from build123d import *

# Parameters (mm, degrees)
SKETCH_1_W          = 20
SKETCH_1_H          = 60
EXTRUDE_1_DEPTH     = 7
SKETCH_4_W          = 30
SKETCH_4_H          = 32
EXTRUDE_2_DEPTH     = 7
SKETCH_3_W          = 9.8
SKETCH_3_H          = 45.5
CUT_EXTRUDE_1_DEPTH = 5
SKETCH_5_W          = 3.5
SKETCH_5_H          = 35
CUT_EXTRUDE_2_DEPTH = 34.911649916
SKETCH_6_R          = 1.1
CUT_EXTRUDE_3_DEPTH = 34.911649916
SKETCH_7_R          = 1.15
CUT_EXTRUDE_4_DEPTH = 35.263683398
FILLET_1_R          = 3
SKETCH_8_R          = 1.95
CUT_EXTRUDE_5_DEPTH = 1


with BuildPart() as part:
    # 草图1 → 凸台-拉伸1 (new body)
    with BuildSketch(Plane(origin=(0, 0, 0), x_dir=(1, 0, 0), z_dir=(0, 1, 0))):
        Rectangle(SKETCH_1_W, SKETCH_1_H)
    extrude(amount=EXTRUDE_1_DEPTH)

    # 草图4 → 凸台-拉伸2 (add)
    with BuildSketch(Plane.XZ):
        with Locations((0, 14)):
            Rectangle(SKETCH_4_W, SKETCH_4_H)
    extrude(amount=-EXTRUDE_2_DEPTH)

    # 草图3 → 切除-拉伸1 (cut)
    with BuildSketch(Plane(origin=(0, 7, 0), x_dir=(1, 0, 0), z_dir=(0, 1, 0))):
        with Locations((0, 2.25)):
            Rectangle(SKETCH_3_W, SKETCH_3_H)
    extrude(amount=-CUT_EXTRUDE_1_DEPTH, mode=Mode.SUBTRACT)

    # 草图5 → 切除-拉伸2 (cut, through all)
    with BuildSketch(Plane(origin=(0, 2, 0), x_dir=(1, 0, 0), z_dir=(0, 1, 0))):
        with Locations((0, 2.25)):
            Rectangle(SKETCH_5_W, SKETCH_5_H)
    extrude(amount=-CUT_EXTRUDE_2_DEPTH, mode=Mode.SUBTRACT)

    # 草图6 → 切除-拉伸3 (cut, through all)
    with BuildSketch(Plane(origin=(0, 2, 0), x_dir=(1, 0, 0), z_dir=(0, 1, 0))):
        with Locations(Location((0, 22.75, 0), (0, 0, 270))):
            Circle(SKETCH_6_R)
        with Locations(Location((0, -18.25, 0), (0, 0, 90))):
            Circle(SKETCH_6_R)
    extrude(amount=-CUT_EXTRUDE_3_DEPTH, mode=Mode.SUBTRACT)

    # 草图7 → 切除-拉伸4 (cut, through all)
    with BuildSketch(Plane(origin=(0, 7, 0), x_dir=(1, 0, 0), z_dir=(0, 1, 0))):
        with Locations(Location((-12, -1, 0), (0, 0, 270))):
            Circle(SKETCH_7_R)
        with Locations(Location((12, -1, 0), (0, 0, 90))):
            Circle(SKETCH_7_R)
        with Locations(Location((12, -27, 0), (0, 0, 270))):
            Circle(SKETCH_7_R)
        with Locations(Location((-12, -27, 0), (0, 0, 90))):
            Circle(SKETCH_7_R)
    extrude(amount=-CUT_EXTRUDE_4_DEPTH, mode=Mode.SUBTRACT)

    # 圆角1
    fillet_1_edges = [part.edges().sort_by_distance(p)[0] for p in [
        (10, 3.5, -2),
        (-10, 3.5, -2),
    ]]
    fillet(fillet_1_edges, radius=FILLET_1_R)

    # 草图8 → 切除-拉伸5 (cut)
    with BuildSketch(Plane.XZ):
        with Locations(Location((0, 18.25, 0), (0, 0, 270))):
            Circle(SKETCH_8_R)
        with Locations(Location((0, -22.75, 0), (0, 0, 270))):
            Circle(SKETCH_8_R)
    extrude(amount=-CUT_EXTRUDE_5_DEPTH, mode=Mode.SUBTRACT)


solid = part.part
CAD build for the part. Positions are in the model's coordinates, mm. A direction names the side the tool comes from. Round coordinates to 2 decimals unless told otherwise and drop trailing zeros. Loops run counter-clockwise (first coordinate to the right, second up) from the corner with the lowest first, then second, coordinate; pieces in that order, holes last. Notation, with made-up numbers: (53, -36) - (106, -36) arc R19 ccw to (106, -9) - close; hole circle Ø4 at (83.25, -31.75). An arc over 180 degrees is marked (long way). Put each result on its own line as item: value.
1. Slice it at B-B on x = 0. List the corners of the cut face in (y, z), and give its area (3 significant figures).
Geometry check:
outline: (0, -30) - (7, -30) - (7, -25) - (2, -25) - (2, -23.85) - (1, -23.85) - (1, -24.7) - (0, -24.7) - close; (0, -20.8) - (1, -20.8) - (1, -21.65) - (2, -21.65) - (2, -19.75) - (0, -19.75) - close; (0, 15.25) - (2, 15.25) - (2, 17.15) - (1, 17.15) - (1, 16.3) - (0, 16.3) - close; (0, 20.2) - (1, 20.2) - (1, 19.35) - (2, 19.35) - (2, 20.5) - (7, 20.5) - (7, 30) - (0, 30) - close
area: 110 mm²
2. Slice it at C-C on y = 3.25. List the corners of the cut face in (x, z).
Geometry check:
outline: (-15, -2) - (-13, -2) arc R3 cw to (-10, -5) - (-10, -30) - (10, -30) - (10, -5) arc R3 cw to (13, -2) - (15, -2) - (15, 30) - (-15, 30) - close; hole circle Ø2.3 at (-12, 1); hole circle Ø2.3 at (-12, 27); hole (-4.9, -25) - (4.9, -25) - (4.9, 20.5) - (-4.9, 20.5) - close; hole circle Ø2.3 at (12, 1); hole circle Ø2.3 at (12, 27)
3. Pin check, flat tip, straight feed: P1, Ø3, axis at x = 0, z = 18.25, coming from the -Y side. Stop position of the tip, or through.
Geometry check:
P1: y = 1
4. 3-axis set-ups, long thin cutter, end or side, ignore diameter. For faces 5 (the flat face through (0, 1, -19.75)), 6 (the flat face through (-1, 1, -24)), 7 (the flat face through (-4.9, 5, -2)), 8 (the flat face through (0, 3, 30)): which of +Z, -Z, +X, -X, +Y, -Y reach the whole face in a straight line?
Geometry check:
face 5: +Y, -Y
face 6: -Y
face 7: +Y
face 8: +Z, +X, -X, +Y, -Y
5. Wall check: line 1 (X direction, y = 2.75, z = 27); line 2 (X direction, y = 1.5, z = 1); line 3 (X direction, y = 1.75, z = 5). Give the ranges that are in metal, low to high.
Geometry check:
line 1: -15 to -13.15, -10.85 to 10.85, 13.15 to 15
line 2: -15 to -13.15, -10.85 to -1.75, 1.75 to 10.85, 13.15 to 15
line 3: -15 to -1.75, 1.75 to 15
6. Slice it at A-A on z = 6. List the corners of the cut face in (x, y), and give its area (3 significant figures).
Geometry check:
outline: (-15, 0) - (-1.75, 0) - (-1.75, 2) - (-4.9, 2) - (-4.9, 7) - (-15, 7) - close; (1.75, 0) - (15, 0) - (15, 7) - (4.9, 7) - (4.9, 2) - (1.75, 2) - close
area: 154 mm²
7. Two-plate mould, pull along X, no slides. Class faces 1 (the flat face through (14, 3, -2)), 2 (the cylindrical face through (-10.98, 3.55, 26.47)), 3 (the flat face through (10, 3, -17)), 4 (the flat face through (0, 5, 20.5)): released by +X, released by -X, zero draft, split by the parting line, or undercut.
Geometry check:
face 1: zero draft
face 2: undercut
face 3: released by +X
face 4: undercut
8. Slice it at D-D on z = 27. List the corners of the cut face in (x, y).
Geometry check:
outline: (-15, 0) - (-13.15, 0) - (-13.15, 7) - (-15, 7) - close; (-10.85, 0) - (10.85, 0) - (10.85, 7) - (-10.85, 7) - close; (13.15, 0) - (15, 0) - (15, 7) - (13.15, 7) - close
